Verification items for the finished model (mm, model axes). A direction names the side the tool comes from. Give positions to 0.01 mm unless a question says otherwise; leave off trailing zeros. Loops run counter-clockwise (first coordinate to the right, second up) from the corner with the lowest first, then second, coordinate; pieces in that order, holes last. Notation, with made-up numbers: M 80,31 L 109,31 A22 cw 109,63 Z; hole C -8.75,15 d6. An arc over 180 degrees is marked long. Answer in a Markdown table with one row per item.
```python
from build123d import *

# Parameters (mm, degrees)
PAD_DEPTH       = 5
SKETCH001_W     = 15
SKETCH001_H     = 7.5
POCKET_DEPTH    = 541.0024137145
SKETCH004_R     = 3.15
POCKET002_DEPTH = 5.001
POCKET003_DEPTH = 5.001


with BuildPart() as part:
    # Sketch → Pad (new body)
    with BuildSketch(Plane.XY):
        Polygon((0, 102.0780970022), (-97.082039325, 31.5438667271), (-60, -82.5829152283), (60, -82.5829152283), (97.082039325, 31.5438667271), align=None)
    extrude(amount=PAD_DEPTH)

    # Sketch001 → Pocket (cut, through all)
    with BuildSketch(Plane.XY.offset(5)):
        Polygon((-84.9467844094, 40.3606455115), (-72.8115294937, 49.1774242959), (-68.4031401016, 43.1097968381), (-80.5383950172, 34.2930180537), align=None)
        Polygon((-12.1352549156, 93.2613182179), (-7.7268655234, 87.19369076), (-19.8621204391, 78.3769119757), (-24.2705111804, 84.4445384533), align=None)
        Polygon((-92.4467844094, 17.2780189827), (-85.3138605372, 19.5956464405), (-80.6786056215, 5.3297986961), (-87.8115294937, 3.0121712383), align=None)
        Polygon((-69.2705098312, -54.0512197394), (-62.137585959, -51.7335922816), (-57.5023310434, -65.999440026), (-64.6352549156, -68.3170674838), align=None)
        with Locations((-37.5, -78.8329152283)):
            Rectangle(SKETCH001_W, SKETCH001_H)
    pocket = extrude(amount=-POCKET_DEPTH, mode=Mode.SUBTRACT)

    # Mirrored: Pocket across Sketch001 V_Axis
    add(pocket.mirror(Plane(origin=(0, 0, 5), x_dir=(0, 0, 1), z_dir=(1, 0, 0))), mode=Mode.SUBTRACT)

    # Sketch004 → Pocket002 (cut, through all)
    with BuildSketch(Plane(origin=(0, 0, 0), x_dir=(1, 0, 0), z_dir=(0, 0, -1))):
        with Locations((-51.2511655217, 70.5411776272)):
            Circle(SKETCH004_R)
        with Locations((-82.9261277772, -26.9443322471)):
            Circle(SKETCH004_R)
        with Locations((0, -87.19369076)):
            Circle(SKETCH004_R)
        with Locations((82.9261277772, -26.9443322471)):
            Circle(SKETCH004_R)
        with Locations((51.2511655217, 70.5411776272)):
            Circle(SKETCH004_R)
    extrude(amount=-POCKET002_DEPTH, mode=Mode.SUBTRACT)

    # Sketch005 → Pocket003 (cut, through all)
    with BuildSketch(Plane(origin=(0, 0, 0), x_dir=(1, 0, 0), z_dir=(0, 0, -1))):
        Polygon((0, -71.1763975648), (67.6927767104, -21.9947164459), (41.8364367999, 57.5829152283), (-41.8364367999, 57.5829152283), (-67.6927767104, -21.9947164459), align=None)
    extrude(amount=-POCKET003_DEPTH, mode=Mode.SUBTRACT)


solid = part.part
```
Item 1: Sectioned sample at C-C (z = 3.1). State how many separate pieces and enclosed holes the cut face has, and give its area (3 significant figures).
Reported:
| item | result |
|---|---|
| separate pieces | 1 |
| enclosed holes | 6 |
| area | 11,400 mm^2 |
Item 2: Scan lines: L1, parallel to Y at x = -1, z = 2; L2, parallel to Y at x = -8, z = 4.6; L3, parallel to X at y = -23, z = 2.6. Record each from-to range of solid material in increasing order. Write a range as [from, to].
Reported:
| item | result |
|---|---|
| L1 | y = [-82.58, -57.58], [70.45, 84.21], [90.18, 101.35] |
| L2 | y = [-82.58, -57.58], [65.36, 87], [87.57, 96.27] |
| L3 | x = [-79.36, -53.07], [53.07, 79.36] |
Item 3: Tool access check on faces 1 (the flat face through (62.3, -75.5, 2.5)), 2 (the flat face through (-9.96, 90.27, 2.54)), 3 (the flat face through (61.019, -67.142, 2.535)), 4 (the flat face through (-65.754, -52.909, 2.535)). Record the directions out of +Z, -Z, +X, -X, +Y, -Y that give a thin tool (end or side, any length) a straight path to the whole face; none if there is none.
Reported:
| item | result |
|---|---|
| face 1 | +Z, -Z, +X, -Y |
| face 2 | +Z, -Z, -X |
| face 3 | +Z, -Z, +X |
| face 4 | +Z, -Z |
Item 4: Sectioned sample at A-A (y = -33). Record the cut outline in (x, z), and give its area (3 significant figures).
Reported:
| item | result |
|---|---|
| outline | M -76.11,0 L -49.82,0 L -49.82,5 L -76.11,5 Z; M 49.82,0 L 76.11,0 L 76.11,5 L 49.82,5 Z |
| area | 263 mm^2 |
Item 5: Sectioned sample at D-D (y = 76). Record the cut outline in (x, z), and give its area (3 significant figures).
Reported:
| item | result |
|---|---|
| outline | M -35.89,0 L 35.89,0 L 35.89,5 L -35.89,5 Z |
| area | 359 mm^2 |
Item 6: Release check for a two-part mould opening along X. For faces 5 (the flat face through (48.881, 66.564, 2.465)), 6 (the cylindrical face through (-86.073, 26.806, 2.465)), 7 (the flat face through (-70.64, 46.19, 2.54)) record: released by +X, released by -X, zero draft, split by the parting line, or undercut.
Reported:
| item | result |
|---|---|
| face 5 | released by +X |
| face 6 | undercut |
| face 7 | released by -X |
Item 7: Go/stop test with flat-tipped pins: pin 1 (2.5 mm diameter, centred on x = -35.5, z = 2.5, fed in from -Y); pin 2 (2.5 mm diameter, centred on y = -78.5, z = 2, fed in from -X); pin 3 (1.5 mm diameter, centred on y = -77.5, z = 3, fed in from -X); pin 4 (5 mm diameter, centred on x = -82.93, y = 26.94, fed in from +Z). Record where each tip stops, or that it passes through.
Reported:
| item | result |
|---|---|
| pin 1 | stops at y = -75.08 |
| pin 2 | stops at x = -61.73 |
| pin 3 | stops at x = -61.9 |
| pin 4 | passes through |
Item 8: Sectioned sample at B-B (x = 15). Record the cut outline in (y, z).
Reported:
| item | result |
|---|---|
| outline | M -82.58,0 L -57.58,0 L -57.58,5 L -82.58,5 Z; M 60.28,0 L 81.91,0 L 81.91,5 L 60.28,5 Z |
